from build123d import *

# Parameters (mm, degrees)
ESQUISSE3_R             = 2.5
ENL_V_MAT_EXTRU_1_DEPTH = 10


with BuildPart() as part:
    # Esquisse2 → Base-R_volution (revolve)
    with BuildSketch(Plane(origin=(0, 0, 0), x_dir=(0, 0, -1), z_dir=(1, 0, 0)), mode=Mode.PRIVATE) as base_r_volution_sk:
        with BuildLine():
            Line((-63.5, 5), (-73.5, 5))
            Line((-73.5, 5), (-73.5, 4))
            Line((-73.5, 4), (-74.5, 4))
            Line((-74.5, 4), (-77.41039886, 0))
            Line((-77.41039886, 0), (-80.010874707, 0))
            ThreePointArc((-80.010874707, 0), (-79.368414789, 4.192388692), (-77.5, 8))
            Line((-77.5, 8), (-63.5, 8))
            Line((-63.5, 8), (-63.5, 5))
        make_face()
    revolve(base_r_volution_sk.sketch.rotate(Axis((0, 0, 0), (0, 0, 1)), 90), axis=Axis((0, 0, 0), (0, 0, 1)))

    # Esquisse3 → Enl_v. mat.-Extru.1 (cut, symmetric)
    with BuildSketch(Plane(origin=(0, 0, 0), x_dir=(1, 0, 0), z_dir=(0, 1, 0))):
        with Locations(Location((0, -67.5, 0), (0, 0, 270))):
            Circle(ESQUISSE3_R)
    extrude(amount=ENL_V_MAT_EXTRU_1_DEPTH, both=True, mode=Mode.SUBTRACT)


solid = part.part
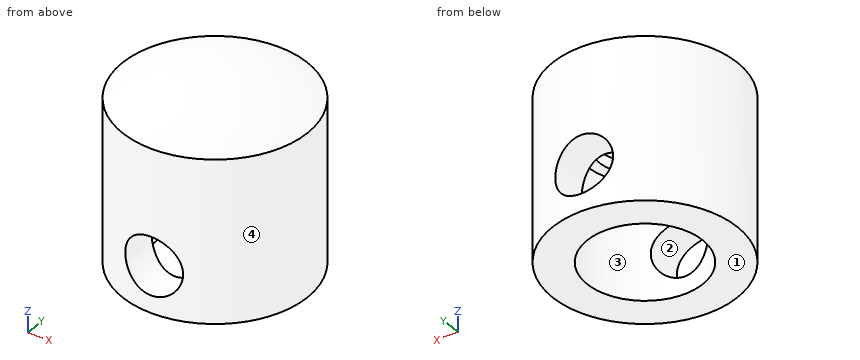
Read the model definition and answer for the solid it produces. Units are mm, in the model's axes. Face numbers are marked on the shaded views. Coordinates: 2 decimals unless noted, no trailing zeros. Write each loop counter-clockwise with the first axis right and the second up, starting at its lowest first coordinate (ties: lowest second). Pieces come first, ordered by that corner, then holes. Notation, with made-up numbers: (-31.75, -36) - (11.25, -36) arc R22 ccw to (11.25, -26) - close; hole circle Ø3 at (-1.5, -22). An arc over 180 degrees is marked (long way). One line per question, with ' | ' between items.
Q1. Find section C-C, the plane x = 0.25. State how many separate pieces and enclosed holes the cut face has, plus the area to 3 significant figures.
Result set:
separate pieces: 3 | enclosed holes: 0 | area: 102 mm^2
Q2. Each of these flat-tipped pins is pushed along its axis until it touches: P1, Ø7, axis at x = 0, y = 0, coming from the -Z side; P2, Ø4, axis at x = 2, y = 3, coming from the +Z side; P3, Ø2, axis at y = 4, z = 72.5, coming from the -X side. Where does it stop, or does it pass through?
Result set:
P1: z = 74.86 | P2: z = 79.92 | P3: x = -7.42
Q3. Find section A-A, the plane z = 67.5. Write down the section's boundary in (x, y).
Result set:
outline: (-2.5, -7.6) - (-2.5, -4.33) arc R5 cw to (-2.5, 4.33) - (-2.5, 7.6) arc R8 ccw to start; (2.5, -7.6) arc R8 ccw to (2.5, 7.6) - (2.5, 4.33) arc R5 cw to (2.5, -4.33) - close
Q4. Consider L1, parallel to Y at x = 0, z = 71.25; L2, parallel to X at y = 1.5, z = 64.5; L3, parallel to X at y = -3.5, z = 67.75. Determine where each line is inside the solid, lowest interval first. Write a range as [from, to].
Result set:
L1: [-8, -5], [5, 8] | L2: [-7.86, -4.77], [4.77, 7.86] | L3: [-7.19, -3.57], [3.57, 7.19]
Q5. Find section B-B, the plane y = -5.5. Write down the section's boundary in (x, z).
Result set:
outline: (-5.81, 63.5) - (5.81, 63.5) - (5.81, 77.5) arc R12.87 ccw to (-5.81, 77.5) - close; hole circle Ø5 at (0, 67.5)
Q6. Find section D-D, the plane z = 73.75. Write down the section's boundary in (x, y).
Result set:
outline: circle Ø16 at (0, 0); hole circle Ø8 at (0, 0)
Q7. Determine the mould class of the marked faces 1, 2, 3 and 4 for opening direction X: +X half, -X half, draft (parallel to the pull), parting line (faces both ways), or undercut.
Result set:
face 1: draft | face 2: undercut | face 3: undercut | face 4: parting line
